Autodesk Inventor part; units mm, degrees
ref_plane "YZ Plane" through (0, 0, 0) normal (1, 0, 0) x (0, 1, 0)
ref_plane "XZ Plane" through (0, 0, 0) normal (0, 1, 0) x (-1, 0, 0)
ref_plane "XY Plane" through (0, 0, 0) normal (0, 0, 1) x (1, 0, 0)
sketch "Sketch1" plane through (0, 0, 0) normal (0, 1, 0) x (-1, 0, 0)
  circle A0 centre (0, 0) radius 4
  circle A1 centre (0, 0) radius 6.5
  dimension "d0" = 8
  dimension "d1" = 13
extrude "Extrusion1" add sketch "Sketch1" along normal blind 8
sketch "Sketch2" plane through (0, 8, 0) normal (0, 1, 0) x (1, 0, 0)
  circle A0 centre (0, 0) radius 20
  dimension "d4" = 40
extrude "Extrusion2" add sketch "Sketch2" along normal blind 5
properties part number "Servo_horn_big"
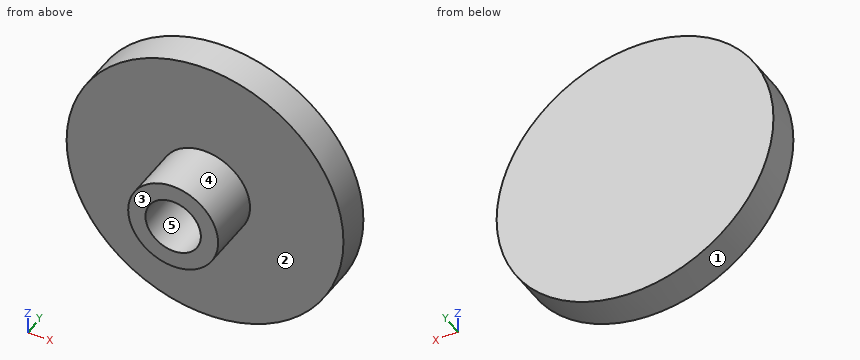
Design review of the part built by this model. Coordinates are the model's own, in mm. Face numbers are marked on the shaded views. A direction names the side the tool comes from. Give positions to 0.01 mm unless a question says otherwise; leave off trailing zeros. Loops run counter-clockwise (first coordinate to the right, second up) from the corner with the lowest first, then second, coordinate; pieces in that order, holes last. Notation, with made-up numbers: (-15.75, 39) -> (42.25, 39) arc R32 ccw to (42.25, 77) -> close; hole circle Ø6 at (42.25, 40.25). An arc over 180 degrees is marked (long way). One line per question, with ' | ' between items. Start each with the question number.
(1) We need section C-C (y = 11.5). State the section outline as (x, z) points.
(2) We need section B-B (z = 0). State the section outline as (x, y) points.
(3) We need section D-D (y = 5.5). State the section outline as (x, z) points.
(4) Insertion check: P1, Ø1, axis at y = 9, z = -3.5, coming from the -X side; P2, Ø5, axis at y = 3.5, z = -2.5, coming from the -X side; P3, Ø1, axis at y = 10, z = 2, coming from the -X side. Each pin has a flat end and moves straight along its axis. Give the tip position at first contact, or say it passes through.
(5) For the marked faces 1 and 2, list the 3-axis set-ups (+Z, -Z, +X, -X, +Y, -Y) from which the entire face can be reached by the end or side of a thin tool; tool diameter is ignored.
(6) We need section A-A (x = 0). State the section outline as (y, z) points, and give its area (3 significant figures).
(7) For line 1 (Z direction, x = 0, y = 2.25); line 2 (Y direction, x = -6, z = 16.5); line 3 (Z direction, x = 1.5, y = 1), list the stretches that pass through material, from the lowest coordinate up.
(8) Draft analysis for pull direction Z (two halves, no side actions). For the marked faces 3, 4 and 5, state which applies: +Z half, -Z half, draft (parallel to the pull), parting line (faces both ways), or undercut.
The answers:
1) outline: circle Ø40 at (0, 0)
2) outline: (-20, 8) -> (-6.5, 8) -> (-6.5, 0) -> (-4, 0) -> (-4, 8) -> (4, 8) -> (4, 0) -> (6.5, 0) -> (6.5, 8) -> (20, 8) -> (20, 13) -> (-20, 13) -> close
3) outline: circle Ø13 at (0, 0); hole circle Ø8 at (0, 0)
4) P1: stops at x = -19.77 | P2: stops at x = -6.5 | P3: stops at x = -19.94
5) face 1: +Y, -Y | face 2: -Y
6) outline: (0, -6.5) -> (8, -6.5) -> (8, -20) -> (13, -20) -> (13, 20) -> (8, 20) -> (8, 6.5) -> (0, 6.5) -> (0, 4) -> (8, 4) -> (8, -4) -> (0, -4) -> close | area: 240 mm^2
7) line 1: z = -6.5 to -4, 4 to 6.5 | line 2: y = 8 to 13 | line 3: z = -6.32 to -3.71, 3.71 to 6.32
8) face 3: draft | face 4: parting line | face 5: undercut
